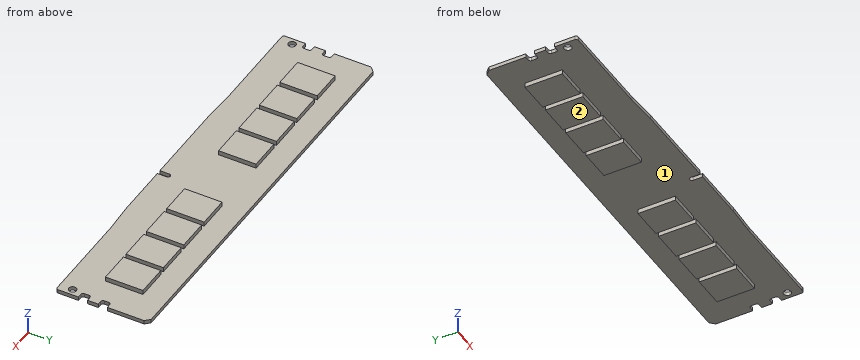
from build123d import *

# Parameters (mm, degrees)
F0_R     = 1.25
F1_DEPTH = 1.27
F2_W     = 10.5
F2_H     = 12.5
F3_DEPTH = 1.5
F4_DEPTH = 2.77


with BuildPart() as f1:
    # F0 (on Top) → F1 (new body)
    with BuildSketch(Plane.XY):
        with BuildLine():
            ThreePointArc((-66.75, -14.45), (-66.53033, -14.98033), (-66, -15.2))
            Line((-66, -15.2), (-34.5, -15.2))
            Line((-34.5, -15.2), (-24.3, -15.7))
            Line((-24.3, -15.7), (4.75, -15.7))
            Line((4.75, -15.7), (4.75, -12.55))
            ThreePointArc((4.75, -12.55), (4.96967, -12.01967), (5.5, -11.8))
            ThreePointArc((5.5, -11.8), (6.03033, -12.01967), (6.25, -12.55))
            Line((6.25, -12.55), (6.25, -15.7))
            Line((6.25, -15.7), (24.3, -15.7))
            Line((24.3, -15.7), (34.5, -15.2))
            Line((34.5, -15.2), (66, -15.2))
            ThreePointArc((66, -15.2), (66.53033, -14.98033), (66.75, -14.45))
            Line((66.75, -14.45), (66.75, -7.7))
            Line((66.75, -7.7), (65.3, -7.7))
            ThreePointArc((65.3, -7.7), (64.76967, -7.48033), (64.55, -6.95))
            Line((64.55, -6.95), (64.55, -5.45))
            ThreePointArc((64.55, -5.45), (64.76967, -4.91967), (65.3, -4.7))
            Line((65.3, -4.7), (66.75, -4.7))
            Line((66.75, -4.7), (66.75, -1.1))
            Line((66.75, -1.1), (65.3, -1.1))
            ThreePointArc((65.3, -1.1), (64.76967, -0.88033), (64.55, -0.35))
            Line((64.55, -0.35), (64.55, 1.15))
            ThreePointArc((64.55, 1.15), (64.76967, 1.68033), (65.3, 1.9))
            Line((65.3, 1.9), (66.75, 1.9))
            Line((66.75, 1.9), (66.75, 14.2))
            Line((66.75, 14.2), (65.25, 15.7))
            Line((65.25, 15.7), (-65.25, 15.7))
            Line((-65.25, 15.7), (-66.75, 14.2))
            Line((-66.75, 14.2), (-66.75, 1.9))
            Line((-66.75, 1.9), (-65.3, 1.9))
            ThreePointArc((-65.3, 1.9), (-64.76967, 1.68033), (-64.55, 1.15))
            Line((-64.55, 1.15), (-64.55, -0.35))
            ThreePointArc((-64.55, -0.35), (-64.76967, -0.88033), (-65.3, -1.1))
            Line((-65.3, -1.1), (-66.75, -1.1))
            Line((-66.75, -1.1), (-66.75, -4.7))
            Line((-66.75, -4.7), (-65.3, -4.7))
            ThreePointArc((-65.3, -4.7), (-64.76967, -4.91967), (-64.55, -5.45))
            Line((-64.55, -5.45), (-64.55, -6.95))
            ThreePointArc((-64.55, -6.95), (-64.76967, -7.48033), (-65.3, -7.7))
            Line((-65.3, -7.7), (-66.75, -7.7))
            Line((-66.75, -7.7), (-66.75, -14.45))
        make_face()
        with Locations((-64.55, -10.9)):
            Circle(F0_R, mode=Mode.SUBTRACT)
        with Locations((64.55, -10.9)):
            Circle(F0_R, mode=Mode.SUBTRACT)
    extrude(amount=F1_DEPTH)

    # F2 (on face) → F3 (join)
    with BuildSketch(Plane.XY.offset(1.27)):
        with Locations((-51.25, 1.75)):
            Rectangle(F2_W, F2_H)
        with Locations((-39.25, 1.75)):
            Rectangle(F2_W, F2_H)
        with Locations((-27.25, 1.75)):
            Rectangle(F2_W, F2_H)
        with Locations((-15.25, 1.75)):
            Rectangle(F2_W, F2_H)
        with Locations((51.25, 1.75)):
            Rectangle(F2_W, F2_H)
        with Locations((39.25, 1.75)):
            Rectangle(F2_W, F2_H)
        with Locations((15.25, 1.75)):
            Rectangle(F2_W, F2_H)
        with Locations((27.25, 1.75)):
            Rectangle(F2_W, F2_H)
    extrude(amount=F3_DEPTH)

    # F2 (on face) → F4 (join)
    with BuildSketch(Plane.XY.offset(1.27)):
        with Locations((-51.25, 1.75)):
            Rectangle(F2_W, F2_H)
        with Locations((-39.25, 1.75)):
            Rectangle(F2_W, F2_H)
        with Locations((-27.25, 1.75)):
            Rectangle(F2_W, F2_H)
        with Locations((-15.25, 1.75)):
            Rectangle(F2_W, F2_H)
        with Locations((51.25, 1.75)):
            Rectangle(F2_W, F2_H)
        with Locations((39.25, 1.75)):
            Rectangle(F2_W, F2_H)
        with Locations((15.25, 1.75)):
            Rectangle(F2_W, F2_H)
        with Locations((27.25, 1.75)):
            Rectangle(F2_W, F2_H)
    extrude(amount=-F4_DEPTH)


solid = f1.part
Model file for the job. Use its own axes, mm. Face numbers are marked on the shaded views. Give positions to 0.01 mm unless a question says otherwise; leave off trailing zeros. Loops run counter-clockwise (first coordinate to the right, second up) from the corner with the lowest first, then second, coordinate; pieces in that order, holes last. Notation, with made-up numbers: (9.5, 18.5) -> (41.5, 18.5) arc R13 cw to (41.5, 24.5) -> close; hole circle Ø1 at (13.5, 15.5). An arc over 180 degrees is marked (long way). Use a Markdown table: item, result. Add a question column.
(1) Mould opens along X. For the marked faces 1 and 2 say: +X half, -X half, draft (parallel to the pull), parting line (faces both ways), or undercut.
(2) Drop flat-ended pins along their axis: pin 1 Ø1.2 at (y, z) = (1.5, -1) entering from -X; pin 2 Ø1 at (y, z) = (-6, 1) entering from -X; pin 3 Ø1.5 at (x, z) = (-41.5, 0.5) entering from -Y. Give the stop position or say it passes through.
(3) Slice it at C-C on x = 49. List the corners of the cut face in (y, z), and give its area (3 significant figures).
(4) Wall check: line 1 along Y through (x, z) = (-58.5, 0.2); line 2 along Z through (x, y) = (-26, 13); line 3 along Y through (x, z) = (55, 2.35). Give the ranges that are in metal, low to high.
(5) Slice it at A-A on x = -17.5. List the corners of the cut face in (y, z).
(6) Slice it at B-B on y = 13. List the corners of the cut face in (x, z).
Filled sheet:
| question | item | result |
|---|---|---|
| 1 | face 1 | undercut |
| 1 | face 2 | draft |
| 2 | pin 1 | x = -56.5 |
| 2 | pin 2 | x = -64.55 |
| 2 | pin 3 | y = -15.2 |
| 3 | outline | (-15.2, 0) -> (-4.5, 0) -> (-4.5, -1.5) -> (8, -1.5) -> (8, 0) -> (15.7, 0) -> (15.7, 1.27) -> (8, 1.27) -> (8, 2.77) -> (-4.5, 2.77) -> (-4.5, 1.27) -> (-15.2, 1.27) -> close |
| 3 | area | 76.7 mm2 |
| 4 | line 1 | -15.2 to 15.7 |
| 4 | line 2 | 0 to 1.27 |
| 4 | line 3 | -4.5 to 8 |
| 5 | outline | (-15.7, 0) -> (-4.5, 0) -> (-4.5, -1.5) -> (8, -1.5) -> (8, 0) -> (15.7, 0) -> (15.7, 1.27) -> (8, 1.27) -> (8, 2.77) -> (-4.5, 2.77) -> (-4.5, 1.27) -> (-15.7, 1.27) -> close |
| 6 | outline | (-66.75, 0) -> (66.75, 0) -> (66.75, 1.27) -> (-66.75, 1.27) -> close |
